from build123d import *

# Parameters (mm, degrees)
F0_R     = 5
F1_DEPTH = 2.5
F3_DEPTH = 1
F4_R     = 0.25


with BuildPart() as f1:
    # F0 (on Top) → F1 (new body)
    with BuildSketch(Plane.XY):
        Circle(F0_R)
    extrude(amount=F1_DEPTH)

    # F2 (on face) → F3 (cut)
    with BuildSketch(Plane.XY.offset(2.5)):
        Polygon((-2.8145825623, -1.625), (0, -3.25), (2.8145825623, -1.625), (2.8145825623, 1.625), (0, 3.25), (-2.8145825623, 1.625), align=None)
    extrude(amount=-F3_DEPTH, mode=Mode.SUBTRACT)

    # F4
    f4_edges = [f1.edges().sort_by_distance(p)[0] for p in [
        (-1.407291, -2.4375, 1.5),
        (1.407291, -2.4375, 1.5),
        (2.814583, 0, 1.5),
        (1.407291, 2.4375, 1.5),
        (-1.407291, 2.4375, 1.5),
        (-2.814583, 0, 1.5),
        (2.814583, -1.625, 2),
        (2.814583, 1.625, 2),
        (2.814583, 0, 2.5),
        (-1.407291, 2.4375, 2.5),
        (-2.814583, 0, 2.5),
        (-2.814583, -1.625, 2),
        (0, -3.25, 2),
        (-1.407291, -2.4375, 2.5),
        (1.407291, -2.4375, 2.5),
        (-5, 0, 2.5),
        (1.407291, 2.4375, 2.5),
    ]]
    fillet(f4_edges, radius=F4_R)


solid = f1.part
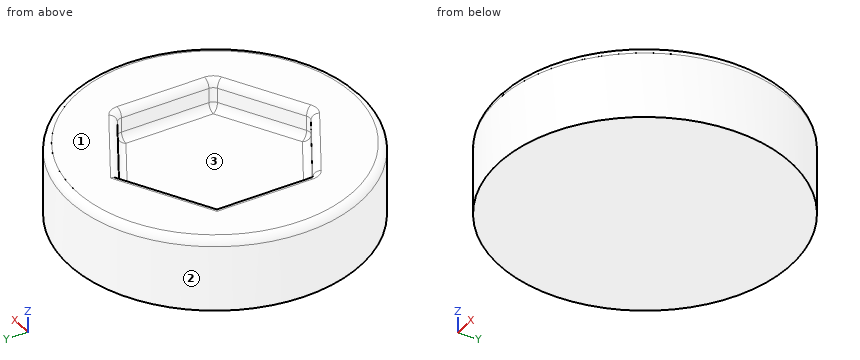
Geometry: final body of the model. Coordinates: model frame, mm. Face numbers are marked on the shaded views. Give positions to 0.01 mm unless a question says otherwise; leave off trailing zeros. Loops run counter-clockwise (first coordinate to the right, second up) from the corner with the lowest first, then second, coordinate; pieces in that order, holes last. Notation, with made-up numbers: (45, -38.5) -> (97, -38.5) arc R36 ccw to (97, 0.5) -> close; hole circle Ø7 at (44.5, 81). An arc over 180 degrees is marked (long way). Put each result on its own line as item: value.
1. Pin query (flat end, axial travel): P1, Ø1, axis at x = 2, z = 2, coming from the +Y side; P2, Ø2.5, axis at x = 0.5, y = 1, coming from the +Z side; P3, Ø0.6, axis at y = -0.5, z = 2, coming from the -X side. Return the tip coordinate at first contact, or that it passes through.
Taken from the geometry:
P1: stops at y = 4.77
P2: stops at z = 1.5
P3: stops at x = -5
2. Cut plane A-A (y = 0). Return the cut outline in (x, z), plus the area to 3 significant figures.
Taken from the geometry:
outline: (-5, 0) -> (5, 0) -> (5, 2.25) arc R0.25 ccw to (4.75, 2.5) -> (3.06, 2.5) arc R0.25 ccw to (2.81, 2.25) -> (2.81, 1.75) arc R0.25 cw to (2.56, 1.5) -> (-2.56, 1.5) arc R0.25 cw to (-2.81, 1.75) -> (-2.81, 2.25) arc R0.25 ccw to (-3.06, 2.5) -> (-4.75, 2.5) arc R0.25 ccw to (-5, 2.25) -> close
area: 19.3 mm2
3. Ray query, line 1 along Z through (x, y) = (-1, -1); line 2 along Z through (x, y) = (3.5, 3.25); line 3 along Y through (x, z) = (0.25, 1.9). Return the intervals inside material, ascending. Write a range as [from, to].
Taken from the geometry:
line 1: z = [0, 1.5]
line 2: z = [0, 2.5]
line 3: y = [-4.99, -3.11], [3.11, 4.99]
4. Pull-direction query (Y, two-part tool) for the marked faces 1, 2 and 3; classes: released by +Y, released by -Y, zero draft, split by the parting line, or undercut.
Taken from the geometry:
face 1: zero draft
face 2: split by the parting line
face 3: undercut
5. Cut plane B-B (z = 1.1). Return the cut outline in (x, y), plus the area to 3 significant figures.
Taken from the geometry:
outline: circle Ø10 at (0, 0)
area: 78.5 mm2
